The listing builds one solid part. Answer for the finished solid, in the listing's coordinates (mm). A direction names the side the tool comes from. Round coordinates to 2 decimals unless told otherwise and drop trailing zeros. Order: outer loops, then holes, each group sorted by start corner. A loop starts at its lowest first (then second) coordinate and runs counter-clockwise, first axis right, second up. Notation, with made-up numbers: (89, -24.5) - (138, -24.5) arc R15 ccw to (138, -14.5) - close; hole circle Ø7 at (20, 86.25). An arc over 180 degrees is marked (long way). One line per item, written item: value. Start each with the question number.
1. Section B-B, the plane y = 46.25 is taken. Give the vertices of the cut face in (x, z).
2. Straight lines are drawn through the part: line 1 (Z direction, x = 0, y = 33); line 2 (Y direction, x = 0, z = 29); line 3 (X direction, y = 60.5, z = 114.75). For each, find the intervals that lie inside material, in ascending order.
3. For a pull along Z with two mould halves and no side action, classify faces 5 (the flat face through (25, 61, 95)), 6 (the flat face through (7, 50, 125.75)), 7 (the flat face through (-12.6, 20.28, 34.89)), 8 (the cylindrical face through (20.33, 61.22, 112.27)) as released by +Z, released by -Z, zero draft, split by the parting line, or undercut.
4. Section C-C, the plane y = -23.75 is taken. Give the vertices of the cut face in (x, z).
5. Section D-D, the plane y = 0 is taken. Count the separate pieces of the cut face and the enclosed holes in it, then the cut area to 3 significant figures.
6. A tool of negligible diameter and unlimited length cuts with its end or side. For faces 1 (the flat face through (0, 61, 69.75)), 2 (the flat face through (5.3, 22.75, 37)), 3 (the cylindrical face through (-6.08, 38.31, 114.16)), 4 (the flat face through (-11.5, 58.75, 88.8)), from which of +Z, -Z, +X, -X, +Y, -Y can it reach the whole face along a straight path? Write none if from no direction.
7. Flat-ended cylindrical pins translate along their axes: P1, Ø1.5, axis at x = -0.5, y = 60.5, coming from the -Z side; P2, Ø2.5, axis at x = -7.5, y = 62.5, coming from the +Z side; P3, Ø1, axis at x = -16, z = 40.5, coming from the +Y side; P4, Ø3, axis at x = 22.5, y = 9.5, coming from the -Z side. Find the tip coordinate at first contact, or state that the pin passes through.
8. Section A-A, the plane z = 42.75 is taken. Give the vertices of the cut face in (x, y), then the cut area to 3 significant figures.
from build123d import *

# Parameters (mm, degrees)
SKETCH1_R                = 12.5
SKETCH1_R_2              = 10
BOSS_EXTRUDE1_START      = -5
SKETCH3_R                = 28.75
SKETCH3_R_2              = 10
BOSS_EXTRUDE1_DEPTH      = 5
HOLE1_D                  = 5
HOLE1_DEPTH              = 5
CIRPATTERN1_COUNT        = 4
SKETCH8_W                = 50
SKETCH8_H                = 50
SKETCH8_R                = 10
BOSS_EXTRUDE3_DEPTH      = 5
FILLET1_R                = 5
HOLE2_D                  = 5
SKETCH11_R               = 7.5
BOSS_EXTRUDE4_DEPTH      = 5
BOSS_EXTRUDE5_REACH      = 135.487
BOSS_EXTRUDE5_END_RADIUS = 12.5
SKETCH12_R               = 10
CUT_EXTRUDE1_REACH       = 135.487
CUT_EXTRUDE1_END_RADIUS  = 10
SKETCH15_R               = 7.5
HOLE4_D                  = 5
BOSS_EXTRUDE6_REACH      = 145.888
BOSS_EXTRUDE6_END_RADIUS = 12.5
SKETCH19_R               = 10
SKETCH19_R_2             = 7.5


with BuildPart() as part:
    # Sweep1: sweep along a path in Sketch2
    with BuildLine(Plane(origin=(0, 0, 0), x_dir=(0, 0, -1), z_dir=(1, 0, 0))) as sweep1_path:
        Line((0, 0), (-76, 0))
        ThreePointArc((-76, 0), (-89.258252147, 5.491747853), (-94.75, 18.75))
        Line((-94.75, 18.75), (-94.75, 63.75))
    # Sketch1 → Sweep1 (sweep)
    with BuildSketch(Plane.XY):
        Circle(SKETCH1_R)
        Circle(SKETCH1_R_2, mode=Mode.SUBTRACT)
    sweep(path=sweep1_path.line)

    # Sketch3 → Boss-Extrude1 (add)
    with BuildSketch(Plane(origin=(0, 0, 0), x_dir=(-1, 0, 0), z_dir=(0, 0, -1)).offset(BOSS_EXTRUDE1_START)):
        Circle(SKETCH3_R)
        with Locations(Location((0, 0, 0), (0, 0, 180))):
            Circle(SKETCH3_R_2, mode=Mode.SUBTRACT)
    extrude(amount=BOSS_EXTRUDE1_DEPTH)

    # Hole1
    with Locations(Plane.XY.offset(5)):
        with Locations((23.75, 0)):
            hole1 = Hole(HOLE1_D / 2, depth=HOLE1_DEPTH)

    # CirPattern1: Hole1 ×4 about axis
    cirpattern1_axis = Axis((0, 0, 0), (0, 0, 1))
    for i in range(1, CIRPATTERN1_COUNT):
        add(hole1.rotate(cirpattern1_axis, i * 360 / CIRPATTERN1_COUNT), mode=Mode.SUBTRACT)

    # Sketch8 → Boss-Extrude3 (add)
    with BuildSketch(Plane(origin=(0, 63.75, 0), x_dir=(1, 0, 0), z_dir=(0, 1, 0))):
        with Locations((0, -94.75)):
            Rectangle(SKETCH8_W, SKETCH8_H)
        with Locations(Location((0, -94.75, 0), (0, 0, 270))):
            Circle(SKETCH8_R, mode=Mode.SUBTRACT)
    extrude(amount=-BOSS_EXTRUDE3_DEPTH)

    # Fillet1
    fillet1_edges = [part.edges().sort_by_distance(p)[0] for p in [
        (25, 61.25, 69.75),
        (25, 61.25, 119.75),
        (-25, 61.25, 119.75),
        (-25, 61.25, 69.75),
    ]]
    fillet(fillet1_edges, radius=FILLET1_R)

    # Hole2 (through all)
    with Locations(Plane(origin=(0, 63.75, 0), x_dir=(1, 0, 0), z_dir=(0, 1, 0))):
        with Locations((20, -74.75), (-20, -74.75), (20, -114.75), (-20, -114.75)):
            Hole(HOLE2_D / 2)



with BuildPart() as body_2:
    # Sketch11 → Boss-Extrude4 (new body)
    with BuildSketch(Plane(origin=(0, 22.75, 0), x_dir=(1, 0, 0), z_dir=(0, 1, 0))):
        with BuildLine():
            Line((-19.642857143, -38.232460485), (-5.357142857, -31.456151214))
            ThreePointArc((-5.357142857, -31.456151214), (0, -30.25), (5.357142857, -31.456151214))
            Line((5.357142857, -31.456151214), (19.642857143, -38.232460485))
            ThreePointArc((19.642857143, -38.232460485), (22.5, -42.75), (19.642857143, -47.267539515))
            Line((19.642857143, -47.267539515), (5.357142857, -54.043848786))
            ThreePointArc((5.357142857, -54.043848786), (0, -55.25), (-5.357142857, -54.043848786))
            Line((-5.357142857, -54.043848786), (-19.642857143, -47.267539515))
            ThreePointArc((-19.642857143, -47.267539515), (-22.5, -42.75), (-19.642857143, -38.232460485))
        make_face()
        with Locations(Location((0, -42.75, 0), (0, 0, 270))):
            Circle(SKETCH11_R, mode=Mode.SUBTRACT)
    extrude(amount=-BOSS_EXTRUDE4_DEPTH)


with BuildPart() as part_1:
    add(part.part)

    add(body_2.part)  # Boss-Extrude5 merges body 2
    # Boss-Extrude5: up to this cylinder (the profile starts outside it)
    boss_extrude5_end = Plane(origin=(0, 0, 42.75), z_dir=(0, 0, 1)) * Cylinder(BOSS_EXTRUDE5_END_RADIUS, 296.974, mode=Mode.PRIVATE)
    # Sketch12 → Boss-Extrude5 (add, up to the surface)
    with BuildSketch(Plane(origin=(0, 22.75, 0), x_dir=(1, 0, 0), z_dir=(0, 1, 0)), mode=Mode.PRIVATE) as boss_extrude5_sk1:
        with Locations(Location((0, -42.75, 0), (0, 0, 270))):
            Circle(SKETCH12_R)
    boss_extrude5_tool1 = extrude(boss_extrude5_sk1.sketch, amount=-BOSS_EXTRUDE5_REACH, mode=Mode.PRIVATE) - boss_extrude5_end
    add(boss_extrude5_tool1.solids().sort_by_distance((0, 22.75, 42.75))[0])

    # Cut-Extrude1: up to this cylinder (the profile starts outside it)
    cut_extrude1_end = Plane(origin=(0, 0, 42.75), z_dir=(0, 0, 1)) * Cylinder(CUT_EXTRUDE1_END_RADIUS, 291.974, mode=Mode.PRIVATE)
    # Sketch15 → Cut-Extrude1 (cut, up to the surface)
    with BuildSketch(Plane(origin=(0, 22.75, 0), x_dir=(1, 0, 0), z_dir=(0, 1, 0)), mode=Mode.PRIVATE) as cut_extrude1_sk1:
        with Locations(Location((0, -42.75, 0), (0, 0, 270))):
            Circle(SKETCH15_R)
    cut_extrude1_tool1 = extrude(cut_extrude1_sk1.sketch, amount=-CUT_EXTRUDE1_REACH, mode=Mode.PRIVATE) - cut_extrude1_end
    add(cut_extrude1_tool1.solids().sort_by_distance((0, 22.75, 42.75))[0], mode=Mode.SUBTRACT)

    # Hole4 (through all)
    with Locations(Plane(origin=(0, 22.75, 0), x_dir=(1, 0, 0), z_dir=(0, 1, 0))):
        with Locations((17.5, -42.75), (-17.5, -42.75)):
            Hole(HOLE4_D / 2)

    # Boss-Extrude6: up to this cylinder (the profile starts outside it)
    boss_extrude6_end = Plane(origin=(0, 36.532843, 94.75), z_dir=(0, 1, 0)) * Cylinder(BOSS_EXTRUDE6_END_RADIUS, 317.776, mode=Mode.PRIVATE)
    # Sketch19 → Boss-Extrude6 (add, up to the surface)
    with BuildSketch(Plane(origin=(0, 0, 125.75), x_dir=(-1, 0, 0), z_dir=(0, 0, -1)), mode=Mode.PRIVATE) as boss_extrude6_sk1:
        with Locations(Location((0, 46.25, 0), (0, 0, 90))):
            Circle(SKETCH19_R)
        with Locations(Location((0, 46.25, 0), (0, 0, 270))):
            Circle(SKETCH19_R_2, mode=Mode.SUBTRACT)
    boss_extrude6_tool1 = extrude(boss_extrude6_sk1.sketch, amount=BOSS_EXTRUDE6_REACH, mode=Mode.PRIVATE) - boss_extrude6_end
    add(boss_extrude6_tool1.solids().sort_by_distance((0, 36.532843, 125.75))[0])


solid = part_1.part
Answer list:
1. outline: (-10, 102.25) arc R12.5 ccw (long way) to (10, 102.25) - (10, 125.75) - (7.5, 125.75) - (7.5, 104.75) arc R12.5 ccw to (-7.5, 104.75) - (-7.5, 125.75) - (-10, 125.75) - close; hole circle Ø20 at (0, 94.75)
2. line 1: z = 82.25 to 84.75, 104.75 to 107.25
2. line 2: y = -12.5 to -10, 10 to 12.5
2. line 3: x = -25 to -22.5, -17.5 to 17.5, 22.5 to 25
3. face 5: zero draft
3. face 6: released by +Z
3. face 7: undercut
3. face 8: undercut
4. outline: (-16.2, 0) - (-2.5, 0) - (-2.5, 5) - (-16.2, 5) - close; (2.5, 0) - (16.2, 0) - (16.2, 5) - (2.5, 5) - close
5. separate pieces: 3
5. enclosed holes: 0
5. area: 653 mm²
6. face 1: -Z, +X, -X, +Y
6. face 2: +X, -X, +Y
6. face 3: +Z
6. face 4: none
7. P1: stops at z = 69.75
7. P2: stops at z = 119.75
7. P3: stops at y = 22.75
7. P4: stops at z = 0
8. outline: (-22.5, 17.75) - (-20, 17.75) - (-20, 22.75) - (-22.5, 22.75) - close; (-15, 17.75) - (-10, 17.75) - (-10, 7.5) arc R12.5 ccw (long way) to (10, 7.5) - (10, 17.75) - (15, 17.75) - (15, 22.75) - (7.5, 22.75) - (7.5, 6.61) arc R10 cw (long way) to (-7.5, 6.61) - (-7.5, 22.75) - (-15, 22.75) - close; (20, 17.75) - (22.5, 17.75) - (22.5, 22.75) - (20, 22.75) - close
8. area: 280 mm²
